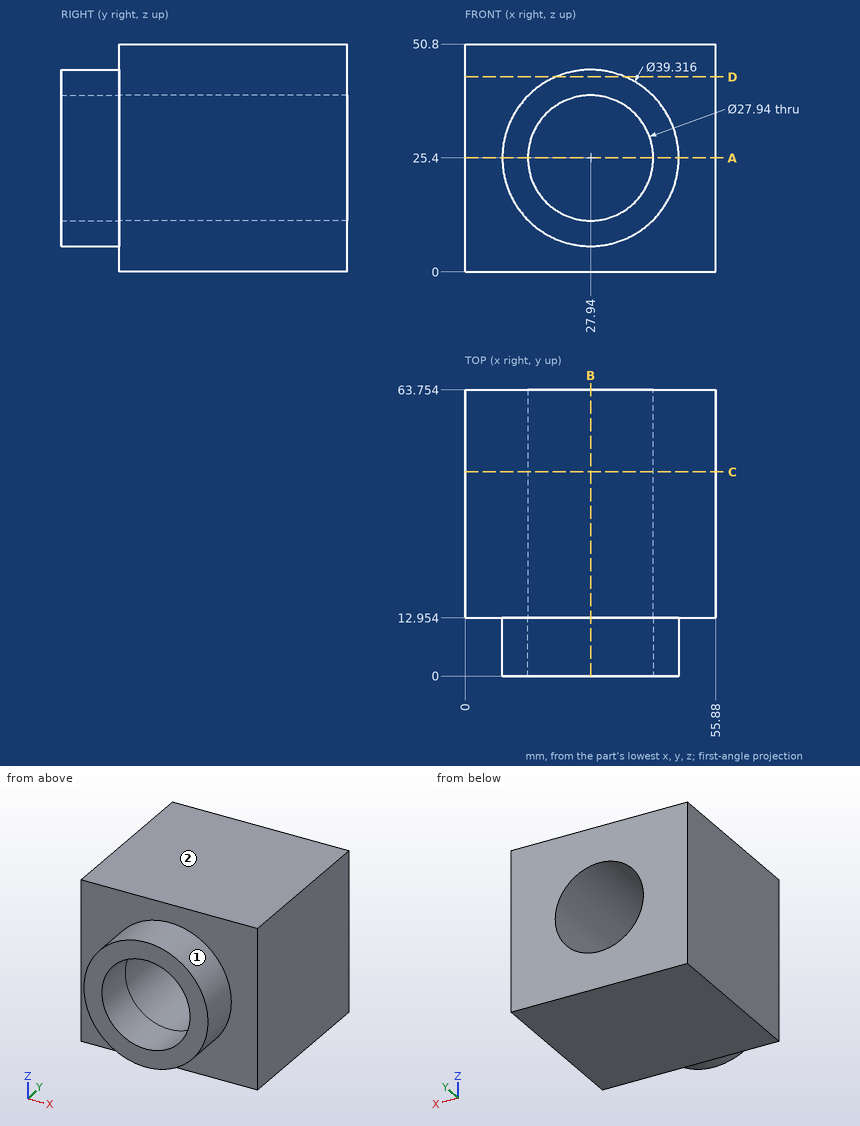
Part print with two shaded views. Sizes in mm from the minimum x, y, z corner. A direction names the side the tool comes from. Round coordinates to 2 decimals unless told otherwise and drop trailing zeros. Loops run counter-clockwise (first coordinate to the right, second up) from the corner with the lowest first, then second, coordinate; pieces in that order, holes last. Notation, with made-up numbers: (39, -39.75) - (69, -39.75) arc R22 cw to (69, -28.75) - close; hole circle Ø1 at (-21.5, 8.25). An arc over 180 degrees is marked (long way). Answer as a JSON object with one key per item and string values.
Item 1: Band-saw the part on A-A on z = 25.4. List the corners of the cut face in (x, y).
Output:
{"outline": "(0, 12.95) - (8.28, 12.95) - (8.28, 0) - (13.97, 0) - (13.97, 63.75) - (0, 63.75) - close; (41.91, 0) - (47.6, 0) - (47.6, 12.95) - (55.88, 12.95) - (55.88, 63.75) - (41.91, 63.75) - close"}
Item 2: Band-saw the part on C-C on y = 45.5. List the corners of the cut face in (x, z).
Output:
{"outline": "(0, 0) - (55.88, 0) - (55.88, 50.8) - (0, 50.8) - close; hole circle Ø27.94 at (27.94, 25.4)"}
Item 3: Band-saw the part on D-D on z = 43.5. List the corners of the cut face in (x, y).
Output:
{"outline": "(0, 12.95) - (20.27, 12.95) - (20.27, 0) - (35.61, 0) - (35.61, 12.95) - (55.88, 12.95) - (55.88, 63.75) - (0, 63.75) - close"}
Item 4: Wall check: L1, parallel to Z at x = 27.94, y = 4.75; L2, parallel to X at y = 3, z = 25 (1 decimal); L3, parallel to Z at x = 27, y = 3 (1 decimal). Give the ranges that are in metal, low to high.
Output:
{"L1": "5.74 to 11.43, 39.37 to 45.06", "L2": "8.3 to 14, 41.9 to 47.6", "L3": "5.8 to 11.5, 39.3 to 45"}
Item 5: Tool access for the marked faces 1 and 2: list every direction of +Z, -Z, +X, -X, +Y, -Y with a clear straight run to the whole face (end or side of a thin tool).
Output:
{"face 1": "-Y", "face 2": "+Z, +X, -X, +Y, -Y"}
Item 6: Band-saw the part on B-B on x = 27.94. List the corners of the cut face in (y, z).
Output:
{"outline": "(0, 5.74) - (12.95, 5.74) - (12.95, 0) - (63.75, 0) - (63.75, 11.43) - (0, 11.43) - close; (0, 39.37) - (63.75, 39.37) - (63.75, 50.8) - (12.95, 50.8) - (12.95, 45.06) - (0, 45.06) - close"}
